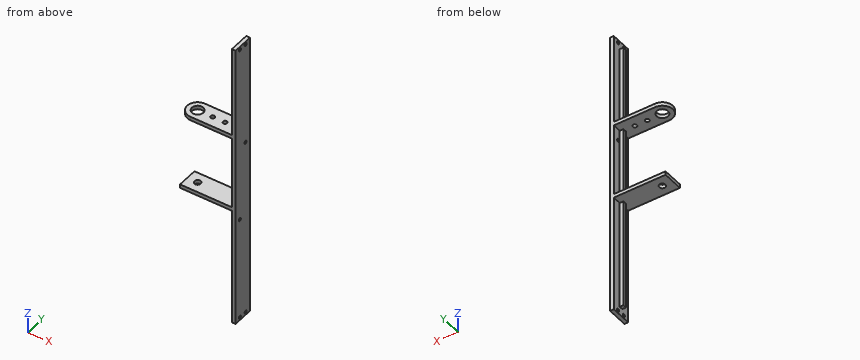
from build123d import *

# Parameters (mm, degrees)
SKETCH_R        = 2.78
SKETCH_R_2      = 1
PAD_DEPTH       = 1.8
SKETCH001_W     = 10
SKETCH001_H     = 140
PAD001_DEPTH    = 1.8
SKETCH002_W     = 10
SKETCH002_H     = 1.8
PAD002_DEPTH    = 25
SKETCH003_R     = 1.5
POCKET_DEPTH    = 82.801
SKETCH004_R     = 0.75
POCKET001_DEPTH = 26.801
SKETCH005_W     = 1.8
SKETCH005_H     = 53.2
SKETCH005_H_2   = 35.2
SKETCH005_H_3   = 40
PAD003_DEPTH    = 1.8


with BuildPart() as part:
    # Sketch → Pad (new body)
    with BuildSketch(Plane.XY):
        with BuildLine():
            ThreePointArc((0, 5), (-5, 0), (0, -5))
            Line((0, -5), (20, -5))
            Line((20, 5), (20, -5))
            Line((0, 5), (20, 5))
        make_face()
        Circle(SKETCH_R, mode=Mode.SUBTRACT)
        with Locations((7.3, 0)):
            Circle(SKETCH_R_2, mode=Mode.SUBTRACT)
        with Locations((13.3, 0)):
            Circle(SKETCH_R_2, mode=Mode.SUBTRACT)
    extrude(amount=PAD_DEPTH)

    # Sketch001 → Pad001 (new body)
    with BuildSketch(Plane.YZ.offset(20)):
        with Locations((0, -24.2)):
            Rectangle(SKETCH001_W, SKETCH001_H)
    extrude(amount=PAD001_DEPTH)

    # Sketch002 → Pad002 (new body)
    with BuildSketch(Plane(origin=(20, 0, 0), x_dir=(0, -1, 0), z_dir=(-1, 0, 0))):
        with Locations((0, -36.1)):
            Rectangle(SKETCH002_W, SKETCH002_H)
    extrude(amount=PAD002_DEPTH)

    # Sketch003 → Pocket (cut, through all)
    with BuildSketch(Plane(origin=(0, 0, -37), x_dir=(1, 0, 0), z_dir=(0, 0, -1))):
        Circle(SKETCH003_R)
    extrude(amount=-POCKET_DEPTH, mode=Mode.SUBTRACT)

    # Sketch004 → Pocket001 (cut, through all)
    with BuildSketch(Plane.YZ.offset(21.8)):
        with Locations((-2, -92.7)):
            Circle(SKETCH004_R)
        with Locations((2, -92.7)):
            Circle(SKETCH004_R)
        with Locations((-2, -42.7)):
            Circle(SKETCH004_R)
        with Locations((2, -5.7)):
            Circle(SKETCH004_R)
        with Locations((2, 44.3)):
            Circle(SKETCH004_R)
        with Locations((-2, 44.3)):
            Circle(SKETCH004_R)
    extrude(amount=-POCKET001_DEPTH, mode=Mode.SUBTRACT)

    # Sketch005 → Pad003 (new body)
    with BuildSketch(Plane(origin=(20, 0, 0), x_dir=(0, -1, 0), z_dir=(-1, 0, 0))):
        with Locations((0, -63.6)):
            Rectangle(SKETCH005_W, SKETCH005_H)
        with Locations((0, -17.6)):
            Rectangle(SKETCH005_W, SKETCH005_H_2)
        with Locations((0, 21.8)):
            Rectangle(SKETCH005_W, SKETCH005_H_3)
    extrude(amount=PAD003_DEPTH)


solid = part.part
Build history of the part. All positions in model axes, mm. Round coordinates to 2 decimals unless told otherwise and drop trailing zeros. Write each loop counter-clockwise with the first axis right and the second up, starting at its lowest first coordinate (ties: lowest second). Pieces come first, ordered by that corner, then holes. Notation, with made-up numbers: M 79,56.5 L 100,56.5 A15 cw 100,75.5 Z; hole C -16.75,22 d4. An arc over 180 degrees is marked long. Answer in a Markdown table with one row per item.
1. Probe L1, parallel to Y at x = 21.3, z = 44.3; L2, parallel to Y at x = 0, z = -36.3; L3, parallel to Z at x = 11.5, y = 4.25. List the from-to ranges inside material, lowest first. Write a range as [from, to].
Geometry check:
| item | result |
|---|---|
| L1 | [-5, -2.75], [-1.25, 1.25], [2.75, 5] |
| L2 | [-5, -1.5], [1.5, 5] |
| L3 | [-37, -35.2], [0, 1.8] |
2. Saw through at B-B (z = 8). List the corners of the cut face in (x, y), and give its area (3 significant figures).
Geometry check:
| item | result |
|---|---|
| outline | M 18.2,-0.9 L 20,-0.9 L 20,-5 L 21.8,-5 L 21.8,5 L 20,5 L 20,0.9 L 18.2,0.9 Z |
| area | 21.2 mm2 |
3. Saw through at A-A (x = 16.75). List the corners of the cut face in (y, z), and give its area (3 significant figures).
Geometry check:
| item | result |
|---|---|
| outline | M -5,-37 L 5,-37 L 5,-35.2 L -5,-35.2 Z; M -5,0 L 5,0 L 5,1.8 L -5,1.8 Z |
| area | 36.0 mm2 |
4. Flat gauge pins, fed straight in: P1, Ø3, axis at x = 15.5, z = -19, coming from the +Y side; P2, Ø1, axis at y = 3, z = -77, coming from the -X side; P3, Ø1.4, axis at y = -0.5, z = -9.5, coming from the -X side; P4, Ø0.5, axis at x = 18.5, y = 0, coming from the -Z side. Where does each tip first touch, or does it go through?
Geometry check:
| item | result |
|---|---|
| P1 | through |
| P2 | x = 20 |
| P3 | x = 18.2 |
| P4 | z = -90.2 |
